Geometry: see drawing. Coordinates: mm, zero at the bounding-box minimum. Round coordinates to 2 decimals unless told otherwise and drop trailing zeros. Loops run counter-clockwise (first coordinate to the right, second up) from the corner with the lowest first, then second, coordinate; pieces in that order, holes last. Notation, with made-up numbers: (-33.75, -0.75) - (4.25, -0.75) arc R14 cw to (4.25, 8.25) - close; hole circle Ø9 at (51, -8.75). An arc over 180 degrees is marked (long way). Return JSON: item names as keys, results as strings. Group by question number.
1. First-contact query: pin 1 Ø2 at (y, z) = (45, 3.1) entering from +X; pin 2 Ø2 at (x, z) = (30, 3.1) entering from -Y. Flat tips, straight axial feed; report the tip coordinate or a pass-through.
2. Material intervals for probe 1 along Z at (x, y) = (10, 3); probe 2 along X at (y, z) = (14.5, 1) (1 decimal); probe 3 along Z at (x, y) = (51, 45), sorted ascending.
3. Section A-A on y = 14. Return loops of the section in (x, z).
4. Section B-B on x = 42. Return loops of the section in (y, z), and give its area (3 significant figures).
5. Section D-D on y = 76. Return loops of the section in (x, z).
6. Section C-C on x = 15. Return loops of the section in (y, z), and give its area (3 significant figures).
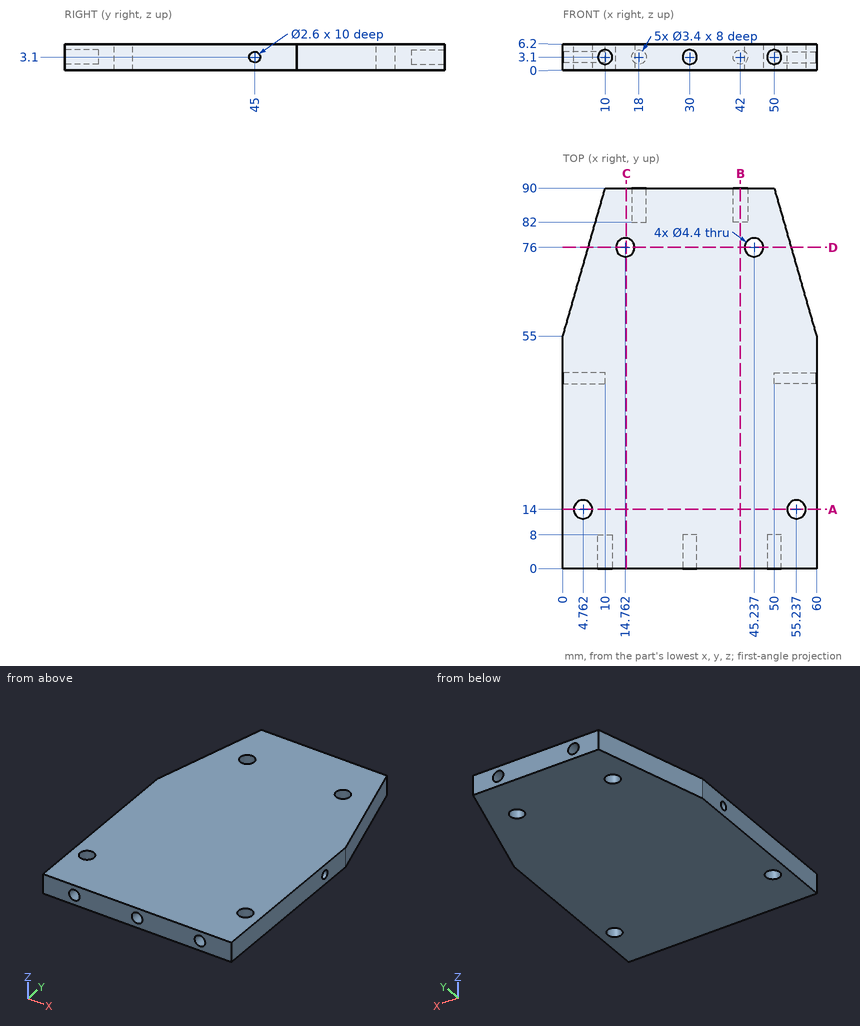
Taken from the geometry:
{
 "1": {"pin 1": "x = 50", "pin 2": "y = 8"},
 "2": {"probe 1": "0 to 1.4, 4.8 to 6.2", "probe 2": "0 to 2.6, 6.9 to 53.1, 57.4 to 60", "probe 3": "0 to 1.8, 4.4 to 6.2"},
 "3": {"outline": "(0, 0) - (2.56, 0) - (2.56, 6.2) - (0, 6.2) - close; (6.96, 0) - (53.04, 0) - (53.04, 6.2) - (6.96, 6.2) - close; (57.44, 0) - (60, 0) - (60, 6.2) - (57.44, 6.2) - close"},
 "4": {"outline": "(0, 0) - (90, 0) - (90, 1.4) - (82, 1.4) - (82, 4.8) - (90, 4.8) - (90, 6.2) - (0, 6.2) - close", "area": "531 mm2"},
 "5": {"outline": "(6, 0) - (12.56, 0) - (12.56, 6.2) - (6, 6.2) - close; (16.96, 0) - (43.04, 0) - (43.04, 6.2) - (16.96, 6.2) - close; (47.44, 0) - (54, 0) - (54, 6.2) - (47.44, 6.2) - close"},
 "6": {"outline": "(0, 0) - (73.81, 0) - (73.81, 6.2) - (0, 6.2) - close; (78.19, 0) - (90, 0) - (90, 6.2) - (78.19, 6.2) - close", "area": "531 mm2"}
}
